Study the drawing (mm; zero at the part's minimum x, y, z) and answer. A direction names the side the tool comes from. Give positions to 0.01 mm unless a question says otherwise; leave off trailing zeros. Loops run counter-clockwise (first coordinate to the right, second up) from the corner with the lowest first, then second, coordinate; pieces in that order, holes last. Notation, with made-up numbers: (85.25, -8.5) - (134.25, -8.5) arc R16 ccw to (134.25, 14.5) - close; hole circle Ø7 at (-17, 28). An arc over 180 degrees is marked (long way). Write item = value, one per line. Start each with the question number.
1) Consider probe 1 along X at (y, z) = (4.75, 7.25); probe 2 along Y at (x, z) = (1.25, 1.75); probe 3 along Y at (x, z) = (0.7, 7). Determine where each line is inside the solid, lowest interval first.
2) The part is cut by section A-A on y = 5.75. Write down the section's boundary in (x, z), plus the area to 3 significant figures.
3) The part is cut by section C-C on x = 1.3. Write down the section's boundary in (y, z), plus the area to 3 significant figures.
4) Which of the six approach directions +Z, -Z, +X, -X, +Y, -Y give full straight-line access (tool end or side, diameter ignored) to the marked faces 5 and 6?
5) The mould has two halves that part along X. Classify the marked faces 1, 2, 3 and 4: +X half, -X half, draft (parallel to the pull), parting line (faces both ways), or undercut.
6) Flat-ended cylindrical pins translate along their axes: P1, Ø1, axis at x = 1.5, y = 4, coming from the -Z side; P2, Ø0.7, axis at x = 1.5, z = 4, coming from the +Y side. Find the tip coordinate at first contact, or state that the pin passes through.
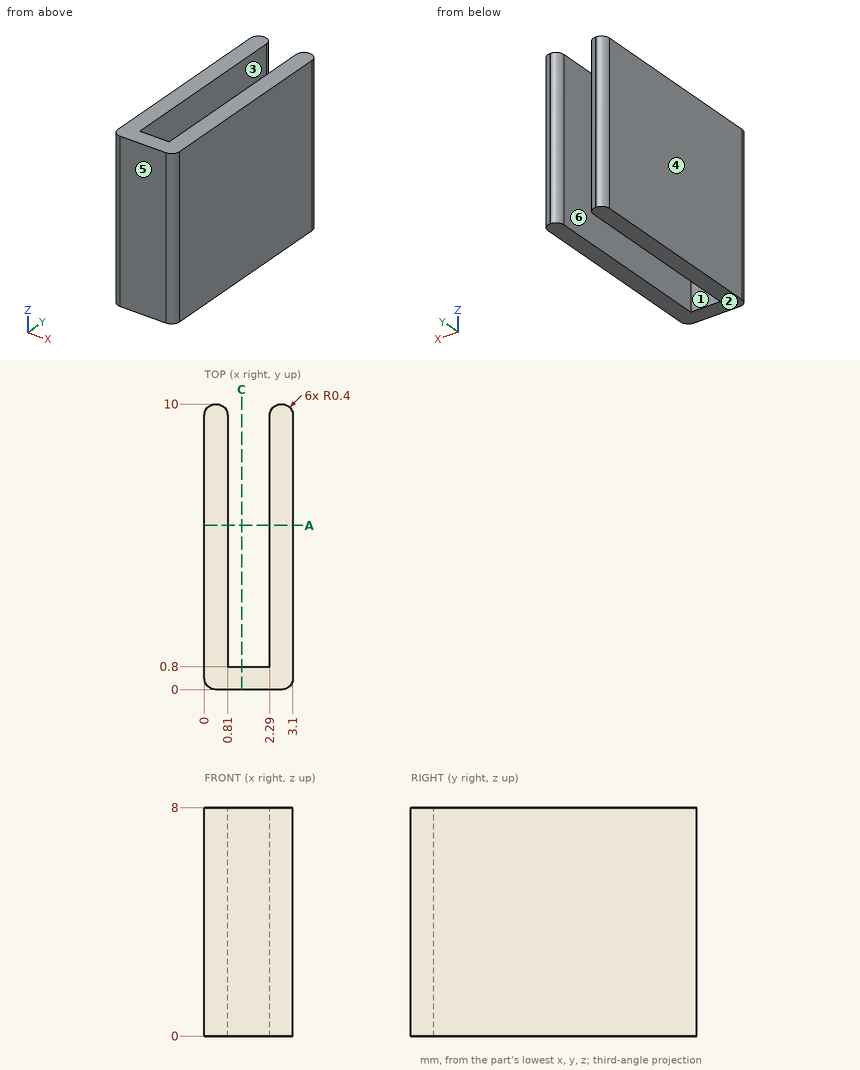
Answer below:
q1.probe_1 = 0 to 0.81, 2.29 to 3.1
q1.probe_2 = 0 to 0.8
q1.probe_3 = 0 to 9.88
q2.outline = (0, 0) - (0.81, 0) - (0.81, 8) - (0, 8) - close; (2.29, 0) - (3.1, 0) - (3.1, 8) - (2.29, 8) - close
q2.area = 13.0 mm2
q3.outline = (0, 0) - (0.8, 0) - (0.8, 8) - (0, 8) - close
q3.area = 6.40 mm2
q4.face_5 = +Z, -Z, +X, -X, -Y
q4.face_6 = +Z, -Z, +Y
q5.face_1 = undercut
q5.face_2 = draft
q5.face_3 = undercut
q5.face_4 = -X half
q6.P1 = through
q6.P2 = 0.8
